```python
from build123d import *

# Parameters (mm, degrees)
BOSS_EXTRUDE2_DEPTH = 25
BOSS_EXTRUDE3_DEPTH = 62.5
BOSS_EXTRUDE5_DEPTH = 62.5


with BuildPart() as part:
    # Sketch1 → Boss-Extrude2 (new body)
    with BuildSketch(Plane.XY):
        with BuildLine():
            ThreePointArc((10.449971294, -17.052803287), (15.972710201, -12.036300463), (19.272609064, -5.344767522))
            Line((19.272609064, -5.344767522), (166.842934549, -32.233408918))
            Line((166.842934549, -32.233408918), (167.478249453, -28.805556447))
            Line((167.478249453, -28.805556447), (19.907923967, -1.91691505))
            ThreePointArc((19.907923967, -1.91691505), (0, 20), (-19.907923967, -1.91691505))
            Line((-19.907923967, -1.91691505), (-167.528286005, -28.529481853))
            Line((-167.528286005, -28.529481853), (-166.892971102, -31.957334324))
            Line((-166.892971102, -31.957334324), (-19.272609064, -5.344767522))
            ThreePointArc((-19.272609064, -5.344767522), (-15.972710201, -12.036300463), (-10.449971294, -17.052803287))
            Line((-10.449971294, -17.052803287), (-76.956361195, -151.503166255))
            Line((-76.956361195, -151.503166255), (-73.836414436, -153.058714328))
            Line((-73.836414436, -153.058714328), (-7.330024534, -18.60835136))
            ThreePointArc((-7.330024534, -18.60835136), (0, -20), (7.330024534, -18.60835136))
            Line((7.330024534, -18.60835136), (74.346110853, -152.805386254))
            Line((74.346110853, -152.805386254), (77.466057613, -151.249838182))
            Line((77.466057613, -151.249838182), (10.449971294, -17.052803287))
        make_face()
        with BuildLine():
            Line((9.838021699, -1.792576093), (19.676043398, -3.585152186))
            ThreePointArc((19.676043398, -3.585152186), (19.670593316, -3.614935491), (19.665098151, -3.64471051))
            Line((19.665098151, -3.64471051), (9.832549076, -1.822355255))
            ThreePointArc((9.832549076, -1.822355255), (7.988292028, -6.015578981), (4.467739088, -8.946468993))
            Line((4.467739088, -8.946468993), (8.935478176, -17.892937986))
            ThreePointArc((8.935478176, -17.892937986), (8.929717682, -17.895813536), (8.923956262, -17.898687232))
            Line((8.923956262, -17.898687232), (4.461978131, -8.949343616))
            ThreePointArc((4.461978131, -8.949343616), (0.015753498, -9.999987591), (-4.433759327, -8.963357531))
            Line((-4.433759327, -8.963357531), (-8.867518653, -17.926715062))
            ThreePointArc((-8.867518653, -17.926715062), (-8.895748496, -17.912723375), (-8.923956262, -17.898687232))
            Line((-8.923956262, -17.898687232), (-4.461978131, -8.949343616))
            ThreePointArc((-4.461978131, -8.949343616), (-7.9863551, -6.018150232), (-9.832549076, -1.822355255))
            Line((-9.832549076, -1.822355255), (-19.665098151, -3.64471051))
            ThreePointArc((-19.665098151, -3.64471051), (-19.67396555, -3.596537162), (-19.682714938, -3.54834224))
            Line((-19.682714938, -3.54834224), (-9.841357469, -1.77417112))
            ThreePointArc((-9.841357469, -1.77417112), (0.009352411, 9.999995627), (9.838021699, -1.792576093))
        make_face(mode=Mode.SUBTRACT)
    extrude(amount=BOSS_EXTRUDE2_DEPTH)

    # Sketch2 → Boss-Extrude3 (add)
    with BuildSketch(Plane.XY.offset(25)):
        Polygon((-167.528286005, -28.529481853), (-19.907923967, -1.91691505), (-19.272609064, -5.344767522), (-166.892971102, -31.957334324), align=None)
    extrude(amount=BOSS_EXTRUDE3_DEPTH)

    # Sketch3 → Boss-Extrude5 (add)
    with BuildSketch(Plane.XY.offset(25)):
        with BuildLine():
            Line((-10.449971294, -17.052803287), (-76.956361195, -151.503166255))
            Line((-76.956361195, -151.503166255), (-73.836414436, -153.058714328))
            Line((-73.836414436, -153.058714328), (-7.330024534, -18.60835136))
            Line((-7.330024534, -18.60835136), (-8.833818914, -17.85858714))
            Line((-8.833818914, -17.85858714), (-8.867518653, -17.926715062))
            ThreePointArc((-8.867518653, -17.926715062), (-8.895748496, -17.912723375), (-8.923956262, -17.898687232))
            Line((-8.923956262, -17.898687232), (-8.889997914, -17.830577323))
            Line((-8.889997914, -17.830577323), (-10.449971294, -17.052803287))
        make_face()
        with BuildLine():
            Line((8.889997914, -17.830577323), (7.330024534, -18.60835136))
            Line((7.330024534, -18.60835136), (74.346110853, -152.805386254))
            Line((74.346110853, -152.805386254), (77.466057613, -151.249838182))
            Line((77.466057613, -151.249838182), (10.449971294, -17.052803287))
            Line((10.449971294, -17.052803287), (8.901477829, -17.824853649))
            Line((8.901477829, -17.824853649), (8.935478176, -17.892937986))
            ThreePointArc((8.935478176, -17.892937986), (8.929717682, -17.895813536), (8.923956262, -17.898687232))
            Line((8.923956262, -17.898687232), (8.889997914, -17.830577323))
        make_face()
        with BuildLine():
            Line((167.478249453, -28.805556447), (19.907923967, -1.91691505))
            Line((19.907923967, -1.91691505), (19.60125996, -3.571525971))
            Line((19.60125996, -3.571525971), (19.676043398, -3.585152186))
            ThreePointArc((19.676043398, -3.585152186), (19.670593316, -3.614935491), (19.665098151, -3.64471051))
            Line((19.665098151, -3.64471051), (19.590266516, -3.630841286))
            Line((19.590266516, -3.630841286), (19.272609064, -5.344767522))
            Line((19.272609064, -5.344767522), (166.842934549, -32.233408918))
            Line((166.842934549, -32.233408918), (167.478249453, -28.805556447))
        make_face()
    extrude(amount=BOSS_EXTRUDE5_DEPTH)


solid = part.part
```
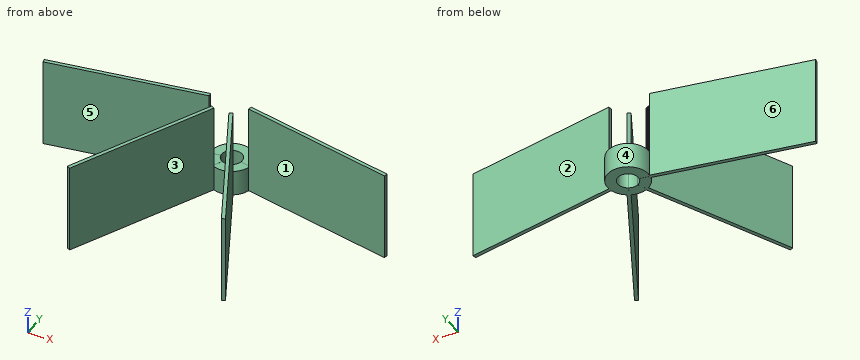
Part model, mm, in its own coordinate system. Face numbers are marked on the shaded views. A direction names the side the tool comes from. Round coordinates to 2 decimals unless told otherwise and drop trailing zeros. Loops run counter-clockwise (first coordinate to the right, second up) from the corner with the lowest first, then second, coordinate; pieces in that order, holes last. Notation, with made-up numbers: (56, -17.5) -> (62, -17.5) arc R11 ccw to (62, -11.5) -> close; hole circle Ø10 at (-37, -7.5). An arc over 180 degrees is marked (long way). Use a Markdown table: item, result.
1) Probe line 1 (X direction, y = 0, z = 16.75); line 2 (X direction, y = -78.5, z = 83); line 3 (Y direction, x = -36.5, z = 46). List the from-to ranges inside material, lowest first. Write a range as [from, to].
The answers:
| item | result |
|---|---|
| line 1 | x = [-20, -10], [10, 20] |
| line 2 | x = [-40.85, -36.96], [37.24, 41.14] |
| line 3 | y = [-77.58, -69.72], [-8.45, -4.91] |
2) Tool access for the marked faces 1 and 2: list every direction of +Z, -Z, +X, -X, +Y, -Y with a clear straight run to the whole face (end or side of a thin tool).
The answers:
| item | result |
|---|---|
| face 1 | +Z, -Z |
| face 2 | +Z, -Z, +X, +Y |
3) Drop flat-ended pins along their axis: pin 1 Ø3.5 at (x, y) = (-1.5, -14.5) entering from +Z; pin 2 Ø4 at (y, z) = (-92.5, 30.5) entering from +X; pin 3 Ø8 at (x, z) = (83, 29) entering from +Y. Give the stop position or say it passes through.
The answers:
| item | result |
|---|---|
| pin 1 | stops at z = 25 |
| pin 2 | stops at x = 49.13 |
| pin 3 | stops at y = -12.68 |
4) Pull direction X, two halves, no side cores. Call the marked faces 3, 4, 5 and 6: pulls with the +X half, pulls with the -X half, needs draft (parallel to the pull), parting line crosses it, or undercut.
The answers:
| item | result |
|---|---|
| face 3 | undercut |
| face 4 | parting line crosses it |
| face 5 | undercut |
| face 6 | pulls with the -X half |
5) Cut at D-D, the plane y = -38. List the corners of the cut face in (x, z), and give its area (3 significant figures).
The answers:
| item | result |
|---|---|
| outline | (-20.81, 0) -> (-16.92, 0) -> (-16.92, 87.5) -> (-20.81, 87.5) -> close; (17.01, 0) -> (20.91, 0) -> (20.91, 87.5) -> (17.01, 87.5) -> close |
| area | 681 mm2 |
6) Cut at B-B, the plane x = -41. List the corners of the cut face in (y, z), and give its area (3 significant figures).
The answers:
| item | result |
|---|---|
| outline | (-86.68, 0) -> (-78.81, 0) -> (-78.81, 87.5) -> (-86.68, 87.5) -> close; (-9.26, 0) -> (-5.72, 0) -> (-5.72, 87.5) -> (-9.26, 87.5) -> close |
| area | 998 mm2 |
7) Cut at A-A, the plane z = 36. State how many separate pieces and enclosed holes the cut face has, and give its area (3 significant figures).
The answers:
| item | result |
|---|---|
| separate pieces | 4 |
| enclosed holes | 0 |
| area | 2,090 mm2 |
